Design review of the part built by this model. Coordinates are the model's own, in mm. A direction names the side the tool comes from. Coordinates: 2 decimals unless noted, no trailing zeros. Write each loop counter-clockwise with the first axis right and the second up, starting at its lowest first coordinate (ties: lowest second). Pieces come first, ordered by that corner, then holes. Notation, with made-up numbers: (-35, 24) -> (-1, 24) arc R13 ccw to (-1, 29) -> close; hole circle Ø2 at (85, -1). An arc over 180 degrees is marked (long way). Answer in a Markdown table with one row per item. Add a question column.
Item 1: For faces 5 (the face through (14, 22, -12)), 6 (the face through (-4, 11, 0)), 7 (the face through (0.51, 8.11, -9.38)), list the 3-axis set-ups (+Z, -Z, +X, -X, +Y, -Y) from which the entire face can be reached by the end or side of a thin tool; tool diameter is ignored.
Item 2: Clearance check with flat-ended pins moving along their axes: P1, Ø6, axis at x = -7.5, y = 22.5, coming from the +Z side; P2, Ø4.5, axis at x = 11, z = 0, coming from the +Y side; P3, Ø5, axis at x = 0, z = 6, coming from the +Y side. State where each tip first meets the part, or that it passes through.
Item 3: Draft analysis for pull direction Z (two halves, no side actions). For faces 1 (the face through (7.15, 66.47, -22.92)), 2 (the face through (-16, 26, -7)), 3 (the face through (-1.978, 5.577, -2.579)), 4 (the face through (2.703, 13.535, 8.584)), state which applies: released by +Z, released by -Z, zero draft, split by the parting line, or undercut.
Item 4: Take a section at C-C, the plane y = 42.5. Write out the cut boundary in (x, z).
Item 5: Take a section at D-D, the plane y = 15. Write out the cut boundary in (x, z).
Item 6: Take a section at B-B, the plane z = 11. Write out the cut boundary in (x, y), and give its area (3 significant figures).
Item 7: To check wall thickness, follow line 1 (X direction, y = 6.25, z = 0); line 2 (X direction, y = 67.5, z = -23.75); line 3 (X direction, y = 8.75, z = -11). State the ranges of each line that lie inside material, in increasing order.
Item 8: Take a section at A-A, the plane x = 0. Write out the cut boundary in (y, z), and give its area (3 significant figures).
from build123d import *

# Parameters (mm, degrees)
SKETCH1_W           = 34
SKETCH1_H           = 34
BOSS_EXTRUDE1_DEPTH = 16
SKETCH2_W           = 34
SKETCH2_H           = 80
BOSS_EXTRUDE2_DEPTH = 12
SKETCH3_R           = 3.25
SKETCH3_R_2         = 1.7
CUT_EXTRUDE2_DEPTH  = 73.291078288
SKETCH4_R           = 9
CUT_EXTRUDE3_DEPTH  = 5
SKETCH5_R           = 1.7
CUT_EXTRUDE4_DEPTH  = 89.572004606
BOSS_EXTRUDE3_DEPTH = 3
BOSS_EXTRUDE4_DEPTH = 3


with BuildPart() as part:
    # Sketch1 → Boss-Extrude1 (new body)
    with BuildSketch(Plane(origin=(0, 0, 0), x_dir=(1, 0, 0), z_dir=(0, 1, 0))):
        Rectangle(SKETCH1_W, SKETCH1_H)
    extrude(amount=BOSS_EXTRUDE1_DEPTH)

    # Sketch2 → Boss-Extrude2 (add)
    with BuildSketch(Plane(origin=(0, 0, -17), x_dir=(-1, 0, 0), z_dir=(0, 0, -1))):
        with Locations((0, 40)):
            Rectangle(SKETCH2_W, SKETCH2_H)
    extrude(amount=BOSS_EXTRUDE2_DEPTH)

    # Sketch3 → Cut-Extrude2 (cut, through all)
    with BuildSketch(Plane(origin=(0, 16, 0), x_dir=(1, 0, 0), z_dir=(0, 1, 0))):
        with Locations(Location((0, 0, 0), (0, 0, 270))):
            Circle(SKETCH3_R)
        with Locations(Location((0, 11, 0), (0, 0, 270))):
            Circle(SKETCH3_R_2)
        with Locations(Location((11, 0, 0), (0, 0, 270))):
            Circle(SKETCH3_R_2)
        with Locations(Location((0, -11, 0), (0, 0, 270))):
            Circle(SKETCH3_R_2)
        with Locations(Location((-11, 0, 0), (0, 0, 270))):
            Circle(SKETCH3_R_2)
    extrude(amount=-CUT_EXTRUDE2_DEPTH, mode=Mode.SUBTRACT)

    # Sketch4 → Cut-Extrude3 (cut)
    with BuildSketch(Plane(origin=(0, 16, 0), x_dir=(1, 0, 0), z_dir=(0, 1, 0))):
        with Locations(Location((0, 0, 0), (0, 0, 270))):
            Circle(SKETCH4_R)
    extrude(amount=-CUT_EXTRUDE3_DEPTH, mode=Mode.SUBTRACT)

    # Sketch5 → Cut-Extrude4 (cut, through all)
    with BuildSketch(Plane.XY.offset(-17)):
        with Locations((-8.5, 67.5)):
            Circle(SKETCH5_R)
        with Locations((8.5, 67.5)):
            Circle(SKETCH5_R)
        with Locations((8.5, 42.5)):
            Circle(SKETCH5_R)
        with Locations((-8.5, 42.5)):
            Circle(SKETCH5_R)
    extrude(amount=-CUT_EXTRUDE4_DEPTH, mode=Mode.SUBTRACT)

    # Sketch6 → Boss-Extrude3 (add)
    with BuildSketch(Plane(origin=(17, 0, 0), x_dir=(0, 0, -1), z_dir=(1, 0, 0))):
        Polygon((17, 16), (-3, 16), (17, 36), align=None)
    extrude(amount=-BOSS_EXTRUDE3_DEPTH)

    # Sketch7 → Boss-Extrude4 (add)
    with BuildSketch(Plane.ZY.offset(17)):
        Polygon((-17, 16), (-17, 36), (3, 16), align=None)
    extrude(amount=-BOSS_EXTRUDE4_DEPTH)


solid = part.part
Answers:
| question | item | result |
|---|---|---|
| 1 | face 5 | +Z, +Y |
| 1 | face 6 | +Y |
| 1 | face 7 | +Y, -Y |
| 2 | P1 | stops at z = -17 |
| 2 | P2 | stops at y = 16 |
| 2 | P3 | stops at y = 11 |
| 3 | face 1 | zero draft |
| 3 | face 2 | released by +Z |
| 3 | face 3 | undercut |
| 3 | face 4 | undercut |
| 4 | outline | (-17, -29) -> (-10.2, -29) -> (-10.2, -17) -> (-17, -17) -> close; (-6.8, -29) -> (6.8, -29) -> (6.8, -17) -> (-6.8, -17) -> close; (10.2, -29) -> (17, -29) -> (17, -17) -> (10.2, -17) -> close |
| 5 | outline | (-17, -29) -> (17, -29) -> (17, 17) -> (-17, 17) -> close; hole circle Ø3.4 at (-11, 0); hole circle Ø18 at (0, 0); hole circle Ø3.4 at (0, -11); hole circle Ø3.4 at (0, 11); hole circle Ø3.4 at (11, 0) |
| 6 | outline | (-17, 0) -> (-1.7, 0) -> (-1.7, 16) -> (-17, 16) -> close; (1.7, 0) -> (17, 0) -> (17, 16) -> (1.7, 16) -> close |
| 6 | area | 490 mm^2 |
| 7 | line 1 | x = -17 to -12.7, -9.3 to -3.25, 3.25 to 9.3, 12.7 to 17 |
| 7 | line 2 | x = -17 to -10.2, -6.8 to 6.8, 10.2 to 17 |
| 7 | line 3 | x = -17 to -1.7, 1.7 to 17 |
| 8 | outline | (0, -29) -> (80, -29) -> (80, -17) -> (16, -17) -> (16, -12.7) -> (0, -12.7) -> close; (0, -9.3) -> (16, -9.3) -> (16, -9) -> (11, -9) -> (11, -3.25) -> (0, -3.25) -> close; (0, 3.25) -> (11, 3.25) -> (11, 9) -> (16, 9) -> (16, 9.3) -> (0, 9.3) -> close; (0, 12.7) -> (16, 12.7) -> (16, 17) -> (0, 17) -> close |
| 8 | area | 1,230 mm^2 |
